The figure shows three views and two pictorial views of one solid part (mm, origin at its lowest corner). Answer the questions. Round coordinates to 2 decimals unless told otherwise and drop trailing zeros. Order: outer loops, then holes, each group sorted by start corner. A loop starts at its lowest first (then second) coordinate and runs counter-clockwise, first axis right, second up. Notation, with made-up numbers: (-16.5, 34) -> (31.5, 34) arc R26 cw to (31.5, 61) -> close; hole circle Ø6 at (-33, 1.5). An arc over 180 degrees is marked (long way). One line per item, written item: value. Start each with the question number.
1. Consider line 1 (Y direction, x = 45, z = 1.6); line 2 (Y direction, x = 31, z = 2.7); line 3 (X direction, y = 21.5, z = 3.6). Determine where each line is inside the solid, lowest interval first.
2. Section D-D (x = 72) is taken. Give the vertices of the cut face in (y, z).
3. Section A-A (x = 45) is taken. Give the vertices of the cut face in (y, z), then the cut area to 3 significant figures.
4. Section C-C (z = 2.55) is taken. State how many separate pieces and enclosed holes the cut face has, then the cut area to 3 significant figures.
5. Section B-B (y = 40) is taken. Give the vertices of the cut face in (x, z), then the cut area to 3 significant figures.
6. Flat-ended cylindrical pins translate along their axes: pin 1 Ø2 at (y, z) = (12, 2) entering from +X; pin 2 Ø1.5 at (x, z) = (88, 3.5) entering from -Y; pin 3 Ø2 at (x, z) = (56.5, 4.5) entering from -Y. Find the tip coordinate at first contact, or state that the pin passes through.
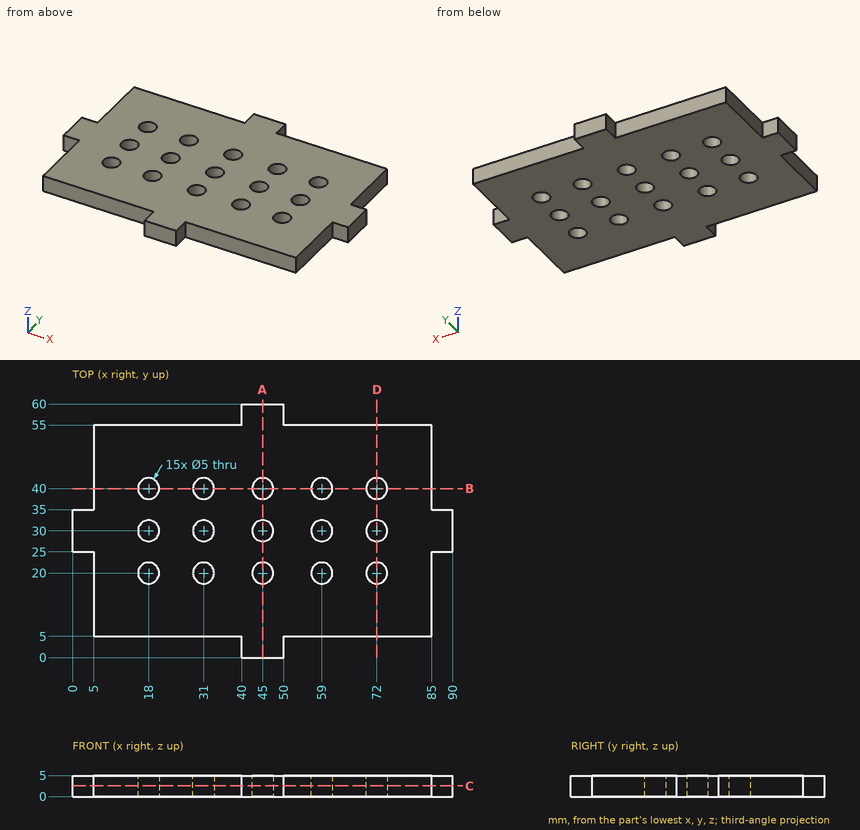
Answer:
1. line 1: 0 to 17.5, 22.5 to 27.5, 32.5 to 37.5, 42.5 to 60
1. line 2: 5 to 17.5, 22.5 to 27.5, 32.5 to 37.5, 42.5 to 55
1. line 3: 5 to 16, 20 to 29, 33 to 43, 47 to 57, 61 to 70, 74 to 85
2. outline: (5, 0) -> (17.5, 0) -> (17.5, 5) -> (5, 5) -> close; (22.5, 0) -> (27.5, 0) -> (27.5, 5) -> (22.5, 5) -> close; (32.5, 0) -> (37.5, 0) -> (37.5, 5) -> (32.5, 5) -> close; (42.5, 0) -> (55, 0) -> (55, 5) -> (42.5, 5) -> close
3. outline: (0, 0) -> (17.5, 0) -> (17.5, 5) -> (0, 5) -> close; (22.5, 0) -> (27.5, 0) -> (27.5, 5) -> (22.5, 5) -> close; (32.5, 0) -> (37.5, 0) -> (37.5, 5) -> (32.5, 5) -> close; (42.5, 0) -> (60, 0) -> (60, 5) -> (42.5, 5) -> close
3. area: 225 mm^2
4. separate pieces: 1
4. enclosed holes: 15
4. area: 3,910 mm^2
5. outline: (5, 0) -> (15.5, 0) -> (15.5, 5) -> (5, 5) -> close; (20.5, 0) -> (28.5, 0) -> (28.5, 5) -> (20.5, 5) -> close; (33.5, 0) -> (42.5, 0) -> (42.5, 5) -> (33.5, 5) -> close; (47.5, 0) -> (56.5, 0) -> (56.5, 5) -> (47.5, 5) -> close; (61.5, 0) -> (69.5, 0) -> (69.5, 5) -> (61.5, 5) -> close; (74.5, 0) -> (85, 0) -> (85, 5) -> (74.5, 5) -> close
5. area: 275 mm^2
6. pin 1: x = 85
6. pin 2: y = 25
6. pin 3: y = 5
